Can you work these out from the model? Positions are in its coordinate system, mm. Face numbers are marked on the shaded views. A direction names the side the tool comes from. Coordinates: 2 decimals unless noted, no trailing zeros. Loops run counter-clockwise (first coordinate to the right, second up) from the corner with the lowest first, then second, coordinate; pieces in that order, holes last.
```python
from build123d import *

# Parameters (mm, degrees)
F0_W      = 23
F0_H      = 12
F1_DEPTH  = 16
F2_W      = 33
F2_H      = 12
F3_DEPTH  = 2
F4_W      = 23
F4_H      = 12
F5_DEPTH  = 6
F7_DEPTH  = 3
F8_R      = 2
F9_DEPTH  = 3
F11_DEPTH = 18.001
F12_R     = 0.5
F13_DEPTH = 3


with BuildPart() as f1:
    # F0 (on Top) → F1 (new body)
    with BuildSketch(Plane.XY):
        Rectangle(F0_W, F0_H)
    extrude(amount=F1_DEPTH)

    # F2 (on face) → F3 (join)
    with BuildSketch(Plane.XY.offset(16)):
        Rectangle(F2_W, F2_H)
    extrude(amount=F3_DEPTH)

    # F4 (on face) → F5 (join)
    with BuildSketch(Plane.XY.offset(18)):
        Rectangle(F4_W, F4_H)
    extrude(amount=F5_DEPTH)

    # F6 (on face) → F7 (join)
    with BuildSketch(Plane.XY.offset(24)):
        with BuildLine():
            ThreePointArc((0.0208333333, -2.4451447071), (6.75, -5.8683472972), (11.5, 0))
            ThreePointArc((11.5, 0), (6.75, 5.8683472972), (0.0208333333, 2.4451447071))
            ThreePointArc((0.0208333333, 2.4451447071), (1.4432039694, 1.572882174), (2, 0))
            ThreePointArc((2, 0), (1.4432039694, -1.572882174), (0.0208333333, -2.4451447071))
        make_face()
        with BuildLine():
            ThreePointArc((2, 0), (1.4432039694, 1.572882174), (0.0208333333, 2.4451447071))
            ThreePointArc((0.0208333333, 2.4451447071), (-0.5, 0), (0.0208333333, -2.4451447071))
            ThreePointArc((0.0208333333, -2.4451447071), (1.4432039694, -1.572882174), (2, 0))
        make_face()
        with BuildLine():
            ThreePointArc((0.0208333333, -2.4451447071), (-0.5, 0), (0.0208333333, 2.4451447071))
            ThreePointArc((0.0208333333, 2.4451447071), (-3, 0), (0.0208333333, -2.4451447071))
        make_face()
    extrude(amount=F7_DEPTH)

    # F8 (on face) → F9 (join)
    with BuildSketch(Plane.XY.offset(27)):
        with Locations((5.5, 0)):
            Circle(F8_R)
    extrude(amount=F9_DEPTH)

    # F10 (on face) → F11 (cut, through all)
    with BuildSketch(Plane.XY.offset(18)):
        with BuildLine():
            ThreePointArc((-15, -0.75), (-13.6047152925, -1.1858541226), (-12.75, 0))
            ThreePointArc((-12.75, 0), (-13.6047152925, 1.1858541226), (-15, 0.75))
            Line((-15, 0.75), (-15, -0.75))
        make_face()
        with BuildLine():
            Line((-15, -0.75), (-15, 0.75))
            ThreePointArc((-15, 0.75), (-15.25, 0), (-15, -0.75))
        make_face()
        with BuildLine():
            ThreePointArc((-15, -0.75), (-15.25, 0), (-15, 0.75))
            Line((-15, 0.75), (-16.5, 0.75))
            Line((-16.5, 0.75), (-16.5, -0.75))
            Line((-16.5, -0.75), (-15, -0.75))
        make_face()
        with BuildLine():
            ThreePointArc((15, -0.75), (15.1858541226, -0.3952847075), (15.25, 0))
            ThreePointArc((15.25, 0), (15.1858541226, 0.3952847075), (15, 0.75))
            Line((15, 0.75), (15, -0.75))
        make_face()
        with BuildLine():
            ThreePointArc((15, 0.75), (15.1858541226, 0.3952847075), (15.25, 0))
            ThreePointArc((15.25, 0), (15.1858541226, -0.3952847075), (15, -0.75))
            Line((15, -0.75), (16.5, -0.75))
            Line((16.5, -0.75), (16.5, 0.75))
            Line((16.5, 0.75), (15, 0.75))
        make_face()
        with BuildLine():
            Line((15, -0.75), (15, 0.75))
            ThreePointArc((15, 0.75), (12.75, 0), (15, -0.75))
        make_face()
    extrude(amount=-F11_DEPTH, mode=Mode.SUBTRACT)

    # F12 (on face) → F13 (cut)
    with BuildSketch(Plane.XY.offset(30)):
        with Locations((5.5, 0)):
            Circle(F12_R)
    extrude(amount=-F13_DEPTH, mode=Mode.SUBTRACT)


solid = f1.part
```
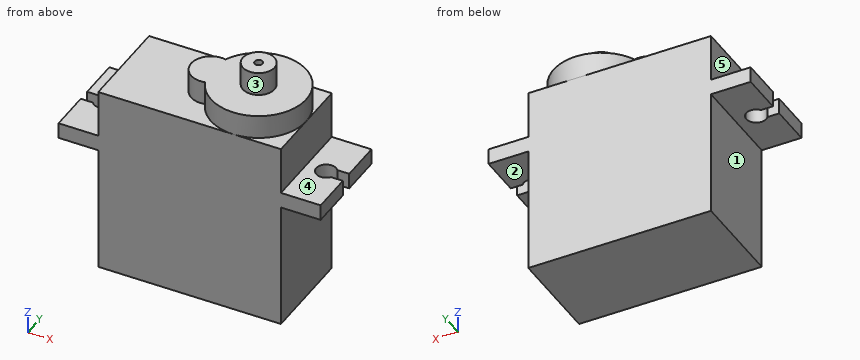
(1) I want a section at C-C on z = 6.5. Write out the boundary of the cut face in (x, y), then the cut area to 3 significant figures.
Check values:
outline: (-11.5, -6) - (11.5, -6) - (11.5, 6) - (-11.5, 6) - close
area: 276 mm2
(2) I want a section at B-B on y = 4.5. Write out the boundary of the cut face in (x, z), then the cut area to 3 significant figures.
Check values:
outline: (-16.5, 16) - (-11.5, 16) - (-11.5, 0) - (11.5, 0) - (11.5, 16) - (16.5, 16) - (16.5, 18) - (11.5, 18) - (11.5, 24) - (9.47, 24) - (9.47, 27) - (1.53, 27) - (1.53, 24) - (-11.5, 24) - (-11.5, 18) - (-16.5, 18) - close
area: 596 mm2
(3) I want a section at D-D on x = 10.5. Write out the boundary of the cut face in (y, z), then the cut area to 3 significant figures.
Check values:
outline: (-6, 0) - (6, 0) - (6, 24) - (3.32, 24) - (3.32, 27) - (-3.32, 27) - (-3.32, 24) - (-6, 24) - close
area: 308 mm2
(4) If I drill on probe 1 along Y at (x, z) = (5.5, 28.2); probe 2 along Y at (x, z) = (14, 16.65); probe 3 along Z at (x, y) = (13, 5.5), over which ranges is the centre line in solid material (lowest first)?
Check values:
probe 1: y = -2 to -0.5, 0.5 to 2
probe 2: y = -6 to -1.25, 1.25 to 6
probe 3: z = 16 to 18
(5) Which directions (+Z, -Z, +X, -X, +Y, -Y) give clear straight access to the entire face, cutting with the end or side of a thin tool? Please do the marked faces 1, 2, 3, 4 and 5.
Check values:
face 1: -Z, -X, +Y, -Y
face 2: -Z, +X, +Y, -Y
face 3: +Z
face 4: +Z, +X, +Y, -Y
face 5: +Z, -X, +Y, -Y
(6) I want a section at A-A on x = -0.5. Write out the boundary of the cut face in (y, z).
Check values:
outline: (-6, 0) - (6, 0) - (6, 24) - (2.5, 24) - (2.5, 27) - (-2.5, 27) - (-2.5, 24) - (-6, 24) - close
(7) I'm going to push flat-ended pins straight in: pin 1 (1.5 mm diameter, centred on x = -13, y = -0.5, fed in from -Z); pin 2 (2 mm diameter, centred on x = -2, y = -2.5, fed in from +Z); pin 3 (2.5 mm diameter, centred on x = 13, y = 1.5, fed in from +Z). Where does each tip first touch, or does it pass through?
Check values:
pin 1: stops at z = 16
pin 2: stops at z = 27
pin 3: stops at z = 18
